Geometry check sheet. Reference: the model listing, model coordinates, mm. A direction names the side the tool comes from. Coordinates: 2 decimals unless noted, no trailing zeros. Write each loop counter-clockwise with the first axis right and the second up, starting at its lowest first coordinate (ties: lowest second). Pieces come first, ordered by that corner, then holes. Notation, with made-up numbers: (38, 37.25) -> (60, 37.25) arc R27 ccw to (60, 54.25) -> close; hole circle Ø1 at (86, 56.25). An arc over 180 degrees is marked (long way). Answer in a Markdown table with one row per item. Add a question column.
1. Mould release check, pull along Y, two halves, no side actions. Record for faces 5 (the flat face through (-61.238, 11.075, 0.056)), 6 (the flat face through (-30, -1.52, 0)), 7 (the flat face through (23.784, 13.251, 0.056)), 8 (the flat face through (-6, 13, 4)): pulls with the +Y half, pulls with the -Y half, needs draft (parallel to the pull), parting line crosses it, or undercut.
2. Scan lines: L1, parallel to Y at x = 42, z = 2.25; L2, parallel to Y at x = 32.5, z = 1.5; L3, parallel to Y at x = 52.5, z = 1. Record each from-to range of solid material in increasing order. Write a range as from..to.
3. Cross-section at C-C on z = 1. Give the number of separate pieces and of enclosed holes in the cut face, and give its area (3 significant figures).
4. Depth check by flat-ended pin: P1, Ø2.5, axis at x = 39.5, z = -1.5, coming from the +Y side; P2, Ø4, axis at x = 28.5, z = 1.5, coming from the -Y side; P3, Ø2.5, axis at x = -40.5, z = 0, coming from the -Y side. Enter the tip coordinate at first touch or a pass-through.
5. Cross-section at B-B on y = -6. Record the cut outline in (x, z), and give its area (3 significant figures).
6. Cross-section at A-A on x = 0. Record the cut outline in (y, z).
7. Set-up check for faces 1 (the flat face through (-56, 22.634, 0)), 2 (the flat face through (-56, 15.868, 0)), 3 (the flat face through (-27, -8.286, 0)), 4 (the cylindrical face through (-32.231, 21.538, 0.056)): record each of +Z, -Z, +X, -X, +Y, -Y from which the full face is reachable in a straight line by a thin tool's end or side.
```python
from build123d import *

# Parameters (mm, degrees)
F0_R     = 11.1
F1_DEPTH = 4
F2_DEPTH = 4
F3_DEPTH = 4
F4_DEPTH = 4
F5_R     = 0.5
F6_R     = 7
F6_R_2   = 5
F7_DEPTH = 4
F8_R     = 5
F9_DEPTH = 25
F10_R    = 12


# Not quite as in the source:
# - a feature names something its author has since deleted; it is built from what else it names


with BuildPart() as f1:
    # F0 (on Top) → F1 (new body, symmetric)
    with BuildSketch(Plane.XY):
        with BuildLine():
            ThreePointArc((20.944924, -1.519927), (20.986226, -0.760462), (21, 0))
            ThreePointArc((21, 0), (20.598026, 4.089169), (19.407495, 8.021792))
            ThreePointArc((19.407495, 8.021792), (0, 21), (-19.407495, 8.021792))
            ThreePointArc((-19.407495, 8.021792), (-20.732595, 3.340581), (-20.944924, -1.519927))
            ThreePointArc((-20.944924, -1.519927), (-20.403011, -4.971634), (-19.296293, -8.285714))
            ThreePointArc((-19.296293, -8.285714), (-6.345132, -20.018474), (11, -17.888544))
            ThreePointArc((11, -17.888544), (13.82448, -15.807712), (16.263142, -13.285714))
            ThreePointArc((16.263142, -13.285714), (17.95462, -10.891815), (19.296293, -8.285714))
            ThreePointArc((19.296293, -8.285714), (20.403011, -4.971634), (20.944924, -1.519927))
        make_face()
        Circle(F0_R, mode=Mode.SUBTRACT)
        with BuildLine():
            Line((20, -20.736863), (16.263142, -13.285714))
            ThreePointArc((16.263142, -13.285714), (13.82448, -15.807712), (11, -17.888544))
            Line((11, -17.888544), (12, -20.842855))
            Line((12, -20.842855), (20, -20.736863))
        make_face()
    extrude(amount=F1_DEPTH, both=True)

    # F0 (on Top) → F2 (join, symmetric)
    with BuildSketch(Plane.XY):
        with BuildLine():
            Line((21.466717, -1.519927), (20.944924, -1.519927))
            ThreePointArc((20.944924, -1.519927), (20.403011, -4.971634), (19.296293, -8.285714))
            Line((19.296293, -8.285714), (35.296293, -8.285714))
            Line((35.296293, -8.285714), (37.758838, -1.519927))
            Line((37.758838, -1.519927), (21.466717, -1.519927))
        make_face()
    extrude(amount=F2_DEPTH, both=True)

    # F0 (on Top) → F3 (join, symmetric)
    with BuildSketch(Plane.XY):
        with BuildLine():
            ThreePointArc((19.407495, 8.021792), (20.598026, 4.089169), (21, 0))
            ThreePointArc((21, 0), (20.986226, -0.760462), (20.944924, -1.519927))
            Line((20.944924, -1.519927), (21.466717, -1.519927))
            Line((21.466717, -1.519927), (22.552058, -0.223202))
            Line((22.552058, -0.223202), (22.998917, -0.223202))
            Line((22.998917, -0.223202), (47.674407, -0.223202))
            Line((47.674407, -0.223202), (50.136952, 6.542585))
            Line((50.136952, 6.542585), (29.636583, 6.542585))
            Line((29.636583, 6.542585), (28.214928, 6.542585))
            Line((28.214928, 6.542585), (29.28627, 7.822585))
            Line((29.28627, 7.822585), (47.431346, 7.822585))
            Line((47.431346, 7.822585), (60.054694, 7.822585))
            Line((60.054694, 7.822585), (62.517239, 14.588372))
            Line((62.517239, 14.588372), (43.96666, 14.588372))
            Line((43.96666, 14.588372), (34.94914, 14.588372))
            Line((34.94914, 14.588372), (36.020482, 15.868372))
            Line((36.020482, 15.868372), (54.509119, 15.868372))
            Line((54.509119, 15.868372), (62.740314, 15.868372))
            Line((62.740314, 15.868372), (76.458602, 15.868372))
            Line((76.458602, 15.868372), (78.921147, 22.634159))
            Line((78.921147, 22.634159), (31.637842, 22.634159))
            Line((31.637842, 22.634159), (19.407495, 8.021792))
        make_face()
    extrude(amount=F3_DEPTH, both=True)

    # F0 (on Top) → F4 (join, symmetric)
    with BuildSketch(Plane.XY):
        with BuildLine():
            ThreePointArc((20.944924, -1.519927), (20.986226, -0.760462), (21, 0))
            ThreePointArc((21, 0), (20.598026, 4.089169), (19.407495, 8.021792))
            ThreePointArc((19.407495, 8.021792), (0, 21), (-19.407495, 8.021792))
            ThreePointArc((-19.407495, 8.021792), (-20.732595, 3.340581), (-20.944924, -1.519927))
            ThreePointArc((-20.944924, -1.519927), (-20.403011, -4.971634), (-19.296293, -8.285714))
            ThreePointArc((-19.296293, -8.285714), (-6.345132, -20.018474), (11, -17.888544))
            ThreePointArc((11, -17.888544), (13.82448, -15.807712), (16.263142, -13.285714))
            ThreePointArc((16.263142, -13.285714), (17.95462, -10.891815), (19.296293, -8.285714))
            ThreePointArc((19.296293, -8.285714), (20.403011, -4.971634), (20.944924, -1.519927))
        make_face()
        Circle(F0_R, mode=Mode.SUBTRACT)
        with BuildLine():
            ThreePointArc((19.407495, 8.021792), (20.598026, 4.089169), (21, 0))
            ThreePointArc((21, 0), (20.986226, -0.760462), (20.944924, -1.519927))
            Line((20.944924, -1.519927), (21.466717, -1.519927))
            Line((21.466717, -1.519927), (22.552058, -0.223202))
            Line((22.552058, -0.223202), (22.998917, -0.223202))
            Line((22.998917, -0.223202), (47.674407, -0.223202))
            Line((47.674407, -0.223202), (50.136952, 6.542585))
            Line((50.136952, 6.542585), (29.636583, 6.542585))
            Line((29.636583, 6.542585), (28.214928, 6.542585))
            Line((28.214928, 6.542585), (29.28627, 7.822585))
            Line((29.28627, 7.822585), (47.431346, 7.822585))
            Line((47.431346, 7.822585), (60.054694, 7.822585))
            Line((60.054694, 7.822585), (62.517239, 14.588372))
            Line((62.517239, 14.588372), (43.96666, 14.588372))
            Line((43.96666, 14.588372), (34.94914, 14.588372))
            Line((34.94914, 14.588372), (36.020482, 15.868372))
            Line((36.020482, 15.868372), (54.509119, 15.868372))
            Line((54.509119, 15.868372), (62.740314, 15.868372))
            Line((62.740314, 15.868372), (76.458602, 15.868372))
            Line((76.458602, 15.868372), (78.921147, 22.634159))
            Line((78.921147, 22.634159), (31.637842, 22.634159))
            Line((31.637842, 22.634159), (19.407495, 8.021792))
        make_face()
        with BuildLine():
            Line((21.466717, -1.519927), (20.944924, -1.519927))
            ThreePointArc((20.944924, -1.519927), (20.403011, -4.971634), (19.296293, -8.285714))
            Line((19.296293, -8.285714), (35.296293, -8.285714))
            Line((35.296293, -8.285714), (37.758838, -1.519927))
            Line((37.758838, -1.519927), (21.466717, -1.519927))
        make_face()
        with BuildLine():
            ThreePointArc((-20.944924, -1.519927), (-20.732595, 3.340581), (-19.407495, 8.021792))
            Line((-19.407495, 8.021792), (-31.637842, 22.634159))
            Line((-31.637842, 22.634159), (-78.921147, 22.634159))
            Line((-78.921147, 22.634159), (-76.458602, 15.868372))
            Line((-76.458602, 15.868372), (-62.740314, 15.868372))
            Line((-62.740314, 15.868372), (-54.509119, 15.868372))
            Line((-54.509119, 15.868372), (-36.020482, 15.868372))
            Line((-36.020482, 15.868372), (-34.94914, 14.588372))
            Line((-34.94914, 14.588372), (-43.96666, 14.588372))
            Line((-43.96666, 14.588372), (-62.517239, 14.588372))
            Line((-62.517239, 14.588372), (-60.054694, 7.822585))
            Line((-60.054694, 7.822585), (-47.431346, 7.822585))
            Line((-47.431346, 7.822585), (-29.28627, 7.822585))
            Line((-29.28627, 7.822585), (-28.214928, 6.542585))
            Line((-28.214928, 6.542585), (-29.636583, 6.542585))
            Line((-29.636583, 6.542585), (-50.136952, 6.542585))
            Line((-50.136952, 6.542585), (-47.674407, -0.223202))
            Line((-47.674407, -0.223202), (-22.552058, -0.223202))
            Line((-22.552058, -0.223202), (-21.466717, -1.519927))
            Line((-21.466717, -1.519927), (-20.944924, -1.519927))
        make_face()
        with BuildLine():
            ThreePointArc((-19.296293, -8.285714), (-20.403011, -4.971634), (-20.944924, -1.519927))
            Line((-20.944924, -1.519927), (-21.466717, -1.519927))
            Line((-21.466717, -1.519927), (-37.758838, -1.519927))
            Line((-37.758838, -1.519927), (-35.296293, -8.285714))
            Line((-35.296293, -8.285714), (-19.296293, -8.285714))
        make_face()
        with BuildLine():
            Line((20, -20.736863), (16.263142, -13.285714))
            ThreePointArc((16.263142, -13.285714), (13.82448, -15.807712), (11, -17.888544))
            Line((11, -17.888544), (12, -20.842855))
            Line((12, -20.842855), (20, -20.736863))
        make_face()
    extrude(amount=F4_DEPTH, both=True)

    # F5
    f5_edges = [f1.edges().sort_by_distance(p)[0] for p in [
        (-36.020482, 15.868372, 0),
        (-29.28627, 7.822585, 0),
        (-22.552058, -0.223202, 0),
        (-19.296293, -8.285714, 0),
        (-21.466717, -1.519927, 0),
        (-28.214928, 6.542585, 0),
        (-34.94914, 14.588372, 0),
        (-78.921147, 22.634159, 0),
        (-76.458602, 15.868372, 0),
        (-62.517239, 14.588372, 0),
        (-60.054694, 7.822585, 0),
        (-50.136952, 6.542585, 0),
        (-37.758838, -1.519927, 0),
        (-35.296293, -8.285714, 0),
        (-47.674407, -0.223202, 0),
        (78.921147, 22.634159, 0),
        (76.458602, 15.868372, 0),
        (62.517239, 14.588372, 0),
        (60.054694, 7.822585, 0),
        (50.136952, 6.542585, 0),
        (37.758838, -1.519927, 0),
        (35.296293, -8.285714, 0),
        (47.674407, -0.223202, 0),
        (21.466717, -1.519927, 0),
        (28.214928, 6.542585, 0),
        (34.94914, 14.588372, 0),
        (36.020482, 15.868372, 0),
        (29.28627, 7.822585, 0),
        (22.552058, -0.223202, 0),
        (19.296293, -8.285714, 0),
        (20, -20.736863, 0),
        (12, -20.842855, 0),
        (11, -17.888544, 0),
        (16.263142, -13.285714, 0),
    ]]
    fillet(f5_edges, radius=F5_R)

    # F6 (on Top) → F7 (join, symmetric)
    with BuildSketch(Plane.XY):
        with Locations((-80.473438, 19.015618)):
            Circle(F6_R)
        with Locations((-80.473438, 19.015618)):
            Circle(F6_R_2, mode=Mode.SUBTRACT)
    extrude(amount=F7_DEPTH, both=True)

    # F8 (on face) → F9 (cut)
    with BuildSketch(Plane.XY.offset(4)):
        with Locations((-80.473438, 19.015618)):
            Circle(F8_R)
    extrude(amount=-F9_DEPTH, mode=Mode.SUBTRACT)

    # F10
    f10_edges = [f1.edges().sort_by_distance(p)[0] for p in [
        (-31.637842, 22.634159, 0),
        (31.637842, 22.634159, 0),
    ]]
    fillet(f10_edges, radius=F10_R)


solid = f1.part
```
Results found:
| question | item | result |
|---|---|---|
| 1 | face 5 | pulls with the -Y half |
| 1 | face 6 | undercut |
| 1 | face 7 | pulls with the +Y half |
| 1 | face 8 | needs draft |
| 2 | L1 | y = -0.22..6.54, 7.82..14.59, 15.87..22.63 |
| 2 | L2 | y = -8.29..-1.52, -0.22..6.54, 7.82..21.66 |
| 2 | L3 | y = 7.82..14.59, 15.87..22.63 |
| 3 | separate pieces | 1 |
| 3 | enclosed holes | 2 |
| 3 | area | 2,920 mm^2 |
| 4 | P1 | stops at y = 22.63 |
| 4 | P2 | stops at y = -8.29 |
| 4 | P3 | stops at y = -0.22 |
| 5 | outline | (-36.13, -4) -> (-9.34, -4) -> (-9.34, 4) -> (-36.13, 4) -> close; (9.34, -4) -> (36.13, -4) -> (36.13, 4) -> (9.34, 4) -> close |
| 5 | area | 429 mm^2 |
| 6 | outline | (-21, -4) -> (-11.1, -4) -> (-11.1, 4) -> (-21, 4) -> close; (11.1, -4) -> (21, -4) -> (21, 4) -> (11.1, 4) -> close |
| 7 | face 1 | +Z, -Z, +X, +Y |
| 7 | face 2 | +Z, -Z |
| 7 | face 3 | +Z, -Z, -X, -Y |
| 7 | face 4 | +Z, -Z, +Y |
